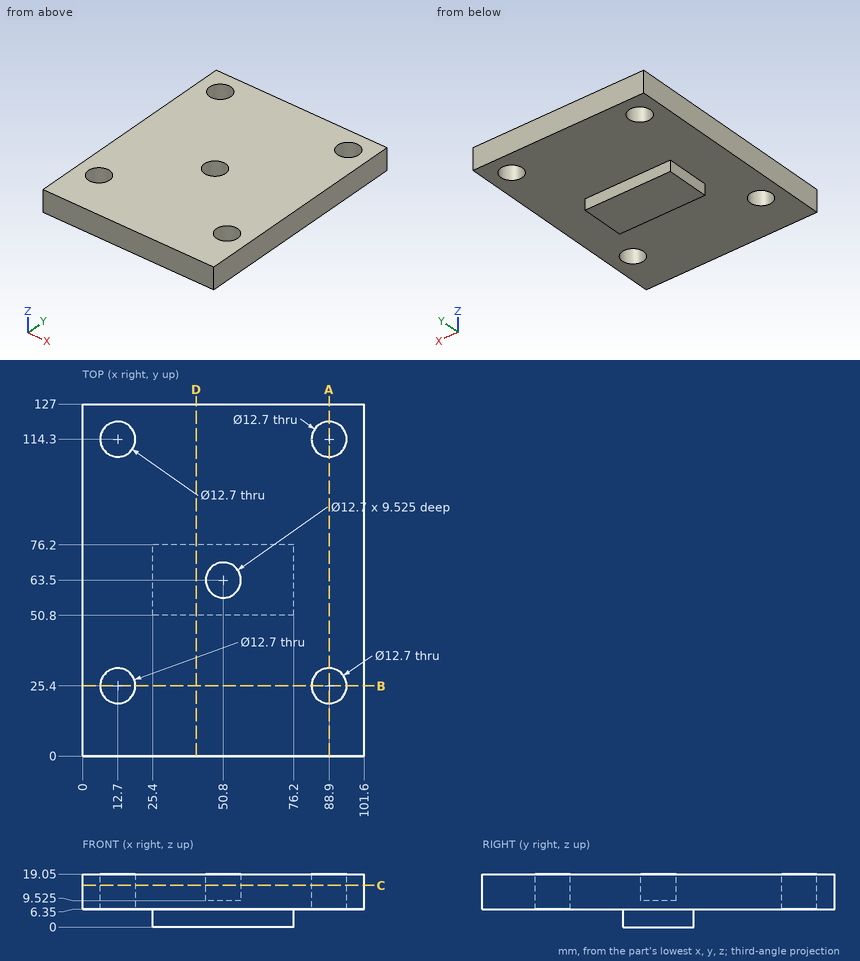
Part print with two shaded views. Sizes in mm from the minimum x, y, z corner. Coordinates: 2 decimals unless noted, no trailing zeros. Loops run counter-clockwise (first coordinate to the right, second up) from the corner with the lowest first, then second, coordinate; pieces in that order, holes last. Notation, with made-up numbers: (-19.5, 79.5) -> (35.5, 79.5) arc R38 cw to (35.5, 118.5) -> close; hole circle Ø6 at (-6.5, 17.25). An arc over 180 degrees is marked (long way). Answer as a JSON object with one key per item and string values.
Q1. Cut at C-C (z = 15). List the corners of the cut face in (x, y), and give its area (3 significant figures).
Report:
{"outline": "(0, 0) -> (101.6, 0) -> (101.6, 127) -> (0, 127) -> close; hole circle Ø12.7 at (12.7, 25.4); hole circle Ø12.7 at (12.7, 114.3); hole circle Ø12.7 at (50.8, 63.5); hole circle Ø12.7 at (88.9, 25.4); hole circle Ø12.7 at (88.9, 114.3)", "area": "12,300 mm2"}
Q2. Cut at A-A (x = 88.9). List the corners of the cut face in (y, z), and give its area (3 significant figures).
Report:
{"outline": "(0, 6.35) -> (19.05, 6.35) -> (19.05, 19.05) -> (0, 19.05) -> close; (31.75, 6.35) -> (107.95, 6.35) -> (107.95, 19.05) -> (31.75, 19.05) -> close; (120.65, 6.35) -> (127, 6.35) -> (127, 19.05) -> (120.65, 19.05) -> close", "area": "1,290 mm2"}
Q3. Flat gauge pins, fed straight in: P1, Ø8, axis at y = 112.5, z = 16.5, coming from the -X side; P2, Ø3, axis at x = 39, z = 4, coming from the -Y side; P3, Ø11.5, axis at x = 12.7, y = 114.3, coming from the -Z side; P4, Ø5, axis at y = 61.5, z = 2.5, coming from the -X side. Where does each tip first touch, or does it go through?
Report:
{"P1": "stops at x = 0", "P2": "stops at y = 50.8", "P3": "passes through", "P4": "stops at x = 25.4"}
Q4. Probe probe 1 along Y at (x, z) = (88.9, 11.25); probe 2 along Y at (x, z) = (50.8, 11.5); probe 3 along Z at (x, y) = (52.5, 67.5) (3 decimals). List the from-to ranges inside material, lowest first.
Report:
{"probe 1": "y = 0 to 19.05, 31.75 to 107.95, 120.65 to 127", "probe 2": "y = 0 to 57.15, 69.85 to 127", "probe 3": "z = 0 to 9.525"}
Q5. Cut at D-D (x = 41). List the corners of the cut face in (y, z).
Report:
{"outline": "(0, 6.35) -> (50.8, 6.35) -> (50.8, 0) -> (76.2, 0) -> (76.2, 6.35) -> (127, 6.35) -> (127, 19.05) -> (0, 19.05) -> close"}
Q6. Cut at B-B (y = 25.4). List the corners of the cut face in (x, z), and give its area (3 significant figures).
Report:
{"outline": "(0, 6.35) -> (6.35, 6.35) -> (6.35, 19.05) -> (0, 19.05) -> close; (19.05, 6.35) -> (82.55, 6.35) -> (82.55, 19.05) -> (19.05, 19.05) -> close; (95.25, 6.35) -> (101.6, 6.35) -> (101.6, 19.05) -> (95.25, 19.05) -> close", "area": "968 mm2"}
